For this review, take the finished solid that the model builds, in its own axes (mm). Face numbers are marked on the shaded views. A direction names the side the tool comes from. Coordinates: 2 decimals unless noted, no trailing zeros. Order: outer loops, then holes, each group sorted by start corner. A loop starts at its lowest first (then second) coordinate and runs counter-clockwise, first axis right, second up. Notation, with made-up numbers: (69, -6.75) - (112, -6.75) arc R20 cw to (112, 30.25) - close; hole circle Ø6 at (-3, 7.25). An arc over 180 degrees is marked (long way). One line per item, written item: value. Start each with the question number.
(1) Clearance check with flat-ended pins moving along their axes: pin 1 (10 mm diameter, centred on x = -7, y = -6.5, fed in from +Z); pin 2 (10 mm diameter, centred on y = -15, z = 3, fed in from -X); pin 3 (1.5 mm diameter, centred on x = -3.5, y = -16.5, fed in from -Z). State where each tip first meets the part, or that it passes through.
(2) Consider section D-D on y = -11.75. Write out the cut boundary in (x, z).
(3) For the marked faces 1 and 2, list the 3-axis set-ups (+Z, -Z, +X, -X, +Y, -Y) from which the entire face can be reached by the end or side of a thin tool; tool diameter is ignored.
(4) Consider section A-A on z = 0. Write out the cut boundary in (x, y).
(5) Consider section B-B on x = 0. Write out the cut boundary in (y, z).
(6) Consider section C-C on y = -17. Write out the cut boundary in (x, z), then the cut area to 3 significant figures.
(7) To check wall thickness, follow line 1 along Z through (x, y) = (0, -18.5); line 2 along Z through (x, y) = (0, -19); line 3 along X through (y, z) = (-15.25, 1.75). State the ranges of each line that lie inside material, in increasing order.
```python
from build123d import *

# Parameters (mm, degrees)
F0_R     = 10.5
F1_DEPTH = 8
F2_R     = 8.4
F3_DEPTH = 0.4
F4_R     = 8.45
F4_R_2   = 8.4
F5_DEPTH = 16
F6_R     = 6.4
F6_R_2   = 5.15
F7_DEPTH = 10
F10_R    = 1


with BuildPart() as f1:
    # F0 (on Front) → F1 (new body)
    with BuildSketch(Plane.XZ):
        Circle(F0_R)
    extrude(amount=F1_DEPTH)

    # F2 (on face) → F3 (join)
    with BuildSketch(Plane.XZ.offset(8)):
        Circle(F2_R)
    extrude(amount=F3_DEPTH)

    # F4 (on face) → F5 (join)
    with BuildSketch(Plane.XZ.offset(8.4)):
        Circle(F4_R)
        Circle(F4_R_2, mode=Mode.SUBTRACT)
        Circle(F4_R_2)
    extrude(amount=F5_DEPTH)

    # F6 (on face) → F7 (cut)
    with BuildSketch(Plane.XZ.offset(24.4)):
        Circle(F6_R)
        Circle(F6_R_2, mode=Mode.SUBTRACT)
    extrude(amount=-F7_DEPTH, mode=Mode.SUBTRACT)

    # F8 (on Right) → F9 (revolve, cut)
    with BuildSketch(Plane.YZ):
        Polygon((-12.4, 8.569138), (-24.4, 8.569138), (-24.4, 6.569138), align=None)
    revolve(axis=Axis((0, -18.4, 0), (0, -1, 0)), mode=Mode.SUBTRACT)

    # F10
    f10_edges = [f1.edges().sort_by_distance(p)[0] for p in [
        (-10.5, -8, 0),
        (-10.5, 0, 0),
    ]]
    fillet(f10_edges, radius=F10_R)


solid = f1.part
```
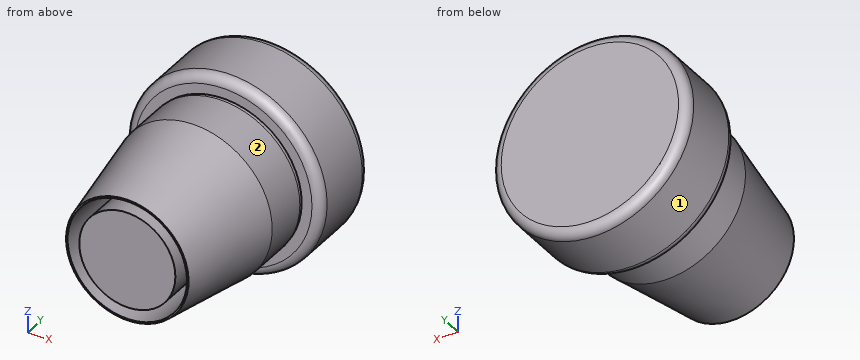
Geometry check:
1. pin 1: stops at z = 10.31
1. pin 2: stops at x = -8.45
1. pin 3: stops at z = -7.42
2. outline: circle Ø16.9 at (0, 0)
3. face 1: +Y, -Y
3. face 2: -Y
4. outline: (-10.5, -7) arc R1 ccw to (-9.5, -8) - (-8.4, -8) - (-8.4, -8.4) - (-8.45, -8.4) - (-8.45, -13.11) - (-6.57, -24.4) - (-6.4, -24.4) - (-6.4, -14.4) - (-5.15, -14.4) - (-5.15, -24.4) - (5.15, -24.4) - (5.15, -14.4) - (6.4, -14.4) - (6.4, -24.4) - (6.57, -24.4) - (8.45, -13.11) - (8.45, -8.4) - (8.4, -8.4) - (8.4, -8) - (9.5, -8) arc R1 ccw to (10.5, -7) - (10.5, -1) arc R1 ccw to (9.5, 0) - (-9.5, 0) arc R1 ccw to (-10.5, -1) - close
5. outline: (-24.4, -6.57) - (-13.11, -8.45) - (-8.4, -8.45) - (-8.4, -8.4) - (-8, -8.4) - (-8, -9.5) arc R1 ccw to (-7, -10.5) - (-1, -10.5) arc R1 ccw to (0, -9.5) - (0, 9.5) arc R1 ccw to (-1, 10.5) - (-7, 10.5) arc R1 ccw to (-8, 9.5) - (-8, 8.4) - (-8.4, 8.4) - (-8.4, 8.45) - (-13.11, 8.45) - (-24.4, 6.57) - (-24.4, 6.4) - (-14.4, 6.4) - (-14.4, 5.15) - (-24.4, 5.15) - (-24.4, -5.15) - (-14.4, -5.15) - (-14.4, -6.4) - (-24.4, -6.4) - close
6. outline: circle Ø15.6 at (0, 0); circle Ø10.3 at (0, 0); hole circle Ø12.8 at (0, 0)
6. area: 146 mm^2
7. line 1: z = -7.55 to -6.4, -5.15 to 5.15, 6.4 to 7.55
7. line 2: z = -7.47 to -6.4, -5.15 to 5.15, 6.4 to 7.47
7. line 3: x = -7.9 to -6.16, -4.84 to 4.84, 6.16 to 7.9
